from build123d import *

# Parameters (mm, degrees)
SKETCH_1_R      = 0.75
EXTRUDE_1_DEPTH = 1


with BuildPart() as part:
    # 草图1 → 凸台-拉伸1 (new body)
    with BuildSketch(Plane(origin=(0, 0, 0), x_dir=(1, 0, 0), z_dir=(0, 1, 0))):
        with BuildLine():
            Line((29.46455474, 22.480687159), (31.403167944, 27.886257161))
            ThreePointArc((31.403167944, 27.886257161), (30.759144982, 30.759144982), (27.886257161, 31.403167944))
            Line((27.886257161, 31.403167944), (22.480687159, 29.46455474))
            ThreePointArc((22.480687159, 29.46455474), (20.287911996, 29.196594839), (18.19369008, 29.899659551))
            ThreePointArc((18.19369008, 29.899659551), (9.447537132, 33.700801803), (0, 35))
            ThreePointArc((0, 35), (-9.447537132, 33.700801803), (-18.19369008, 29.899659551))
            ThreePointArc((-18.19369008, 29.899659551), (-20.287911996, 29.196594839), (-22.480687159, 29.46455474))
            Line((-22.480687159, 29.46455474), (-27.886257161, 31.403167944))
            ThreePointArc((-27.886257161, 31.403167944), (-30.759144982, 30.759144982), (-31.403167944, 27.886257161))
            Line((-31.403167944, 27.886257161), (-29.46455474, 22.480687159))
            ThreePointArc((-29.46455474, 22.480687159), (-29.196594839, 20.287911996), (-29.899659551, 18.19369008))
            ThreePointArc((-29.899659551, 18.19369008), (-33.052834782, 11.511303701), (-34.732884242, 4.315872125))
            Line((-34.732884242, 4.315872125), (-32.190837206, 4))
            ThreePointArc((-32.190837206, 4), (-30.89823255, 3.292285123), (-30.441307179, 1.891247526))
            ThreePointArc((-30.441307179, 1.891247526), (-30.5, 0), (-30.441307179, -1.891247526))
            ThreePointArc((-30.441307179, -1.891247526), (-30.89823255, -3.292285123), (-32.190837206, -4))
            Line((-32.190837206, -4), (-34.732884242, -4.315872125))
            ThreePointArc((-34.732884242, -4.315872125), (-33.052834782, -11.511303701), (-29.899659551, -18.19369008))
            ThreePointArc((-29.899659551, -18.19369008), (-29.196594839, -20.287911996), (-29.46455474, -22.480687159))
            Line((-29.46455474, -22.480687159), (-31.403167944, -27.886257161))
            ThreePointArc((-31.403167944, -27.886257161), (-30.759144982, -30.759144982), (-27.886257161, -31.403167944))
            Line((-27.886257161, -31.403167944), (-22.480687159, -29.46455474))
            ThreePointArc((-22.480687159, -29.46455474), (-20.287911996, -29.196594839), (-18.19369008, -29.899659551))
            ThreePointArc((-18.19369008, -29.899659551), (-9.447537132, -33.700801803), (0, -35))
            ThreePointArc((0, -35), (9.447537132, -33.700801803), (18.19369008, -29.899659551))
            ThreePointArc((18.19369008, -29.899659551), (20.287911996, -29.196594839), (22.480687159, -29.46455474))
            Line((22.480687159, -29.46455474), (27.886257161, -31.403167944))
            ThreePointArc((27.886257161, -31.403167944), (30.759144982, -30.759144982), (31.403167944, -27.886257161))
            Line((31.403167944, -27.886257161), (29.46455474, -22.480687159))
            ThreePointArc((29.46455474, -22.480687159), (29.196594839, -20.287911996), (29.899659551, -18.19369008))
            ThreePointArc((29.899659551, -18.19369008), (33.700801803, -9.447537132), (35, 0))
            ThreePointArc((35, 0), (33.700801803, 9.447537132), (29.899659551, 18.19369008))
            ThreePointArc((29.899659551, 18.19369008), (29.196594839, 20.287911996), (29.46455474, 22.480687159))
        make_face()
        with Locations(Location((-28.814601333, -28.814601333, 0), (0, 0, 270))):
            Circle(SKETCH_1_R, mode=Mode.SUBTRACT)
        with BuildLine():
            Line((-14.476872329, -18.719513016), (-10.868928268, -15.111568955))
            ThreePointArc((-10.868928268, -15.111568955), (-10.22008157, -14.678023452), (-9.454714705, -14.525782517))
            Line((-9.454714705, -14.525782517), (9.454714705, -14.525782517))
            ThreePointArc((9.454714705, -14.525782517), (10.22008157, -14.678023452), (10.868928268, -15.111568955))
            Line((10.868928268, -15.111568955), (14.476872329, -18.719513016))
            ThreePointArc((14.476872329, -18.719513016), (15.051657451, -20.343212221), (14.151213664, -21.811537127))
            ThreePointArc((14.151213664, -21.811537127), (0, -26), (-14.151213664, -21.811537127))
            ThreePointArc((-14.151213664, -21.811537127), (-15.051657451, -20.343212221), (-14.476872329, -18.719513016))
        make_face(mode=Mode.SUBTRACT)
        with BuildLine():
            ThreePointArc((1.828205899, -10.397220329), (2.466819597, -11.815731007), (1.048308919, -12.454344705))
            ThreePointArc((1.048308919, -12.454344705), (-1.042632246, -11.445222173), (-2.926575027, -10.088342356))
            ThreePointArc((-2.926575027, -10.088342356), (-3.041516382, -8.536959591), (-1.490133616, -8.422018236))
            ThreePointArc((-1.490133616, -8.422018236), (0.082632246, -9.554777827), (1.828205899, -10.397220329))
        make_face(mode=Mode.SUBTRACT)
        with Locations(Location((28.814601333, -28.814601333, 0), (0, 0, 270))):
            Circle(SKETCH_1_R, mode=Mode.SUBTRACT)
        with BuildLine():
            ThreePointArc((14.466575027, -10.088342356), (12.582632246, -11.445222173), (10.491691081, -12.454344705))
            ThreePointArc((10.491691081, -12.454344705), (9.073180403, -11.815731007), (9.711794101, -10.397220329))
            ThreePointArc((9.711794101, -10.397220329), (11.457367754, -9.554777827), (13.030133616, -8.422018236))
            ThreePointArc((13.030133616, -8.422018236), (14.581516382, -8.536959591), (14.466575027, -10.088342356))
        make_face(mode=Mode.SUBTRACT)
        with BuildLine():
            Line((-11.97, 6.898932188), (-11.97, -6.898932188))
            ThreePointArc((-11.97, -6.898932188), (-12.122240935, -7.664299053), (-12.555786438, -8.313145751))
            Line((-12.555786438, -8.313145751), (-18.719513016, -14.476872329))
            ThreePointArc((-18.719513016, -14.476872329), (-20.343212221, -15.051657451), (-21.811537127, -14.151213664))
            ThreePointArc((-21.811537127, -14.151213664), (-26, 0), (-21.811537127, 14.151213664))
            ThreePointArc((-21.811537127, 14.151213664), (-20.343212221, 15.051657451), (-18.719513016, 14.476872329))
            Line((-18.719513016, 14.476872329), (-12.555786438, 8.313145751))
            ThreePointArc((-12.555786438, 8.313145751), (-12.122240935, 7.664299053), (-11.97, 6.898932188))
        make_face(mode=Mode.SUBTRACT)
        with BuildLine():
            ThreePointArc((-2.926575027, 10.088342356), (-1.042632246, 11.445222173), (1.048308919, 12.454344705))
            ThreePointArc((1.048308919, 12.454344705), (2.466819597, 11.815731007), (1.828205899, 10.397220329))
            ThreePointArc((1.828205899, 10.397220329), (0.082632246, 9.554777827), (-1.490133616, 8.422018236))
            ThreePointArc((-1.490133616, 8.422018236), (-3.041516382, 8.536959591), (-2.926575027, 10.088342356))
        make_face(mode=Mode.SUBTRACT)
        with Locations(Location((-28.814601333, 28.814601333, 0), (0, 0, 270))):
            Circle(SKETCH_1_R, mode=Mode.SUBTRACT)
        with BuildLine():
            ThreePointArc((10.868928268, 15.111568955), (10.22008157, 14.678023452), (9.454714705, 14.525782517))
            Line((9.454714705, 14.525782517), (-9.454714705, 14.525782517))
            ThreePointArc((-9.454714705, 14.525782517), (-10.22008157, 14.678023452), (-10.868928268, 15.111568955))
            Line((-10.868928268, 15.111568955), (-14.476872329, 18.719513016))
            ThreePointArc((-14.476872329, 18.719513016), (-15.051657451, 20.343212221), (-14.151213664, 21.811537127))
            ThreePointArc((-14.151213664, 21.811537127), (0, 26), (14.151213664, 21.811537127))
            ThreePointArc((14.151213664, 21.811537127), (15.051657451, 20.343212221), (14.476872329, 18.719513016))
            Line((14.476872329, 18.719513016), (10.868928268, 15.111568955))
        make_face(mode=Mode.SUBTRACT)
        with BuildLine():
            ThreePointArc((9.711794101, 10.397220329), (9.073180403, 11.815731007), (10.491691081, 12.454344705))
            ThreePointArc((10.491691081, 12.454344705), (12.582632246, 11.445222173), (14.466575027, 10.088342356))
            ThreePointArc((14.466575027, 10.088342356), (14.581516382, 8.536959591), (13.030133616, 8.422018236))
            ThreePointArc((13.030133616, 8.422018236), (11.457367754, 9.554777827), (9.711794101, 10.397220329))
        make_face(mode=Mode.SUBTRACT)
        with BuildLine():
            ThreePointArc((21.811537127, -14.151213664), (20.343212221, -15.051657451), (18.719513016, -14.476872329))
            Line((18.719513016, -14.476872329), (17.434140759, -13.191500072))
            ThreePointArc((17.434140759, -13.191500072), (17.000595257, -12.542653375), (16.848354322, -11.77728651))
            Line((16.848354322, -11.77728651), (16.848354322, 11.77728651))
            ThreePointArc((16.848354322, 11.77728651), (17.000595257, 12.542653375), (17.434140759, 13.191500072))
            Line((17.434140759, 13.191500072), (18.719513016, 14.476872329))
            ThreePointArc((18.719513016, 14.476872329), (20.343212221, 15.051657451), (21.811537127, 14.151213664))
            ThreePointArc((21.811537127, 14.151213664), (26, 0), (21.811537127, -14.151213664))
        make_face(mode=Mode.SUBTRACT)
        with Locations(Location((28.814601333, 28.814601333, 0), (0, 0, 270))):
            Circle(SKETCH_1_R, mode=Mode.SUBTRACT)
    extrude(amount=EXTRUDE_1_DEPTH)


solid = part.part
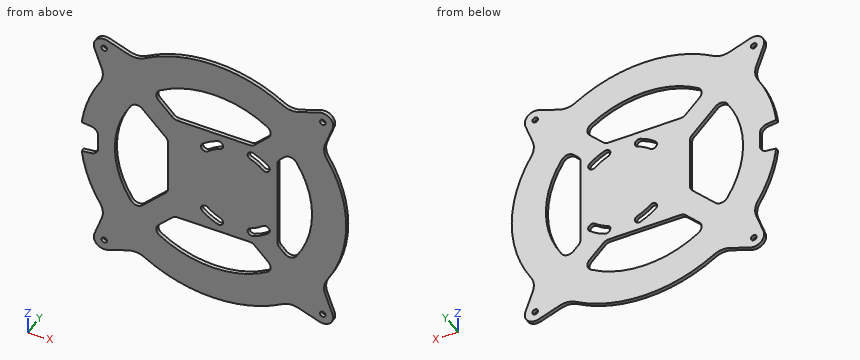
Can you work these out from the model? Positions are in its coordinate system, mm. Coordinates: 2 decimals unless noted, no trailing zeros. Write each loop counter-clockwise with the first axis right and the second up, starting at its lowest first coordinate (ties: lowest second). Pieces come first, ordered by that corner, then holes. Notation, with made-up numbers: (78.25, -33.75) -> (104.25, -33.75) arc R24 ccw to (104.25, -11.75) -> close; hole circle Ø8 at (-40, 73). An arc over 180 degrees is marked (long way). Write each question's results on one line, items separated by ' | '. Start each with the question number.
Item 1: I'm going to push flat-ended pins straight in: P1, Ø1.4, axis at x = 28.81, z = -28.81, coming from the +Y side; P2, Ø0.5, axis at x = -2, y = 0.5, coming from the +Z side; P3, Ø0.5, axis at y = 0.5, z = 1.5, coming from the -X side. Where does each tip first touch, or does it pass through?
Item 2: If we section it at B-B, the plane z = 17: Write out the boundary of the cut face in (x, y).
Item 3: If we section it at C-C, the plane y = 0.55: Count the separate pieces of the cut face and the enclosed holes in it, and give its area (3 significant figures).
Item 4: Please list where these lines run through material, in increasing order: probe 1 along X at (y, z) = (0.8, -5); probe 2 along Z at (x, y) = (12.5, 0.2); probe 3 along Z at (x, y) = (-6.5, 0.6).
Item 5: If we section it at A-A, the plane x = 5: Write out the boundary of the cut face in (y, z), and give its area (3 significant figures).
Answer block:
1) P1: through | P2: z = 34.96 | P3: x = -30.47
2) outline: (-30.59, 0) -> (-12.76, 0) -> (-12.76, 1) -> (-30.59, 1) -> close; (12.76, 0) -> (30.59, 0) -> (30.59, 1) -> (12.76, 1) -> close
3) separate pieces: 1 | enclosed holes: 12 | area: 2,920 mm²
4) probe 1: -34.64 to -25.51, -11.97 to 16.85, 25.51 to 34.64 | probe 2: -32.69 to -22.8, -16.74 to -11.49, -8.85 to 8.85, 11.49 to 16.74, 22.8 to 32.69 | probe 3: -34.39 to -25.17, -14.53 to 14.53, 25.17 to 34.39
5) outline: (0, -34.64) -> (1, -34.64) -> (1, -25.51) -> (0, -25.51) -> close; (0, -14.53) -> (1, -14.53) -> (1, 14.53) -> (0, 14.53) -> close; (0, 25.51) -> (1, 25.51) -> (1, 34.64) -> (0, 34.64) -> close | area: 47.3 mm²
